from build123d import *

# Parameters (mm, degrees)
SM_BASE_FLANGE_1_DEPTH = 100
CUT_EXTRUDE_1_DEPTH    = 102.727577382
PATTERN_LINEAR_6_COUNT = 4
PATTERN_LINEAR_6_PITCH = 25
SKETCH2_W              = 120.770502754
SKETCH2_H              = 115.80541844
CUT_EXTRUDE1_DEPTH     = 15


# Sheet-metal steps are written as plain solids
with BuildPart() as part:
    # Sketch 1 → Базовая кромка1 (new body)
    with BuildSketch(Plane(origin=(0, 0, 0), x_dir=(0, 0, -1), z_dir=(1, 0, 0))):
        with BuildLine():
            Line((-17.5, 6.5), (-14.5, 6.5))
            ThreePointArc((-14.5, 6.5), (-13.792893219, 6.207106781), (-13.5, 5.5))
            Line((-13.5, 5.5), (-13.5, 2))
            ThreePointArc((-13.5, 2), (-12.914213562, 0.585786438), (-11.5, 0))
            Line((-11.5, 0), (11.5, 0))
            ThreePointArc((11.5, 0), (12.914213562, 0.585786438), (13.5, 2))
            Line((13.5, 2), (13.5, 5.5))
            ThreePointArc((13.5, 5.5), (13.792893219, 6.207106781), (14.5, 6.5))
            Line((14.5, 6.5), (17.5, 6.5))
            Line((17.5, 6.5), (17.5, 7.5))
            Line((17.5, 7.5), (14.5, 7.5))
            ThreePointArc((14.5, 7.5), (13.085786438, 6.914213562), (12.5, 5.5))
            Line((12.5, 5.5), (12.5, 2))
            ThreePointArc((12.5, 2), (12.207106781, 1.292893219), (11.5, 1))
            Line((11.5, 1), (-11.5, 1))
            ThreePointArc((-11.5, 1), (-12.207106781, 1.292893219), (-12.5, 2))
            Line((-12.5, 2), (-12.5, 5.5))
            ThreePointArc((-12.5, 5.5), (-13.085786438, 6.914213562), (-14.5, 7.5))
            Line((-14.5, 7.5), (-17.5, 7.5))
            Line((-17.5, 7.5), (-17.5, 6.5))
        make_face()
    extrude(amount=SM_BASE_FLANGE_1_DEPTH)

    # Эскиз6 → Вырез-Вытянуть1 (cut, through all)
    with BuildSketch(Plane(origin=(0, 1, 0), x_dir=(1, 0, 0), z_dir=(0, 1, 0))):
        with BuildLine():
            Line((6.65, 3.15), (18.35, 3.15))
            ThreePointArc((18.35, 3.15), (21.5, 0), (18.35, -3.15))
            Line((18.35, -3.15), (6.65, -3.15))
            ThreePointArc((6.65, -3.15), (3.5, 0), (6.65, 3.15))
        make_face()
    cut_extrude_1 = extrude(amount=-CUT_EXTRUDE_1_DEPTH, mode=Mode.SUBTRACT)

    # Линейный массив6: Вырез-Вытянуть1 ×4
    with Locations(*[(i * PATTERN_LINEAR_6_PITCH, 0, 0) for i in range(1, PATTERN_LINEAR_6_COUNT)]):
        add(cut_extrude_1, mode=Mode.SUBTRACT)

    # Sketch2 → Cut-Extrude1 (cut)
    with BuildSketch(Plane.ZY):
        with Locations((-11.279080545, 0.592045476)):
            Rectangle(SKETCH2_W, SKETCH2_H)
    extrude(amount=-CUT_EXTRUDE1_DEPTH, mode=Mode.SUBTRACT)


solid = part.part
Geometry check sheet. Reference: the model listing, model coordinates, mm. A direction names the side the tool comes from. Round coordinates to 2 decimals unless told otherwise and drop trailing zeros. Order: outer loops, then holes, each group sorted by start corner. A loop starts at its lowest first (then second) coordinate and runs counter-clockwise, first axis right, second up. Notation, with made-up numbers: (1.25, 85.5) - (38.25, 85.5) arc R16 ccw to (38.25, 111.5) - close; hole circle Ø6 at (44, -38.5). An arc over 180 degrees is marked (long way). One line per question, with ' | ' between items. Start each with the question number.
(1) Sectioned sample at D-D on x = 20.5. Record the cut outline in (y, z).
(2) Thickness scan on L1, parallel to Z at x = 68, y = 4; L2, parallel to Y at x = 85.5, z = 8; L3, parallel to Y at x = 63, z = -14.5. Record the ranges inside material, lowest first. Write a range as [from, to].
(3) Sectioned sample at A-A on z = 0. Record the cut outline in (x, y), and give its area (3 significant figures).
(4) Release check for a two-part mould opening along Z. For faces 1 (the cylindrical face through (78.5, 0.5, 0.1)), 2 (the flat face through (57, 4, -12.5)), 3 (the flat face through (57, 6.5, 16)), 4 (the cylindrical face through (56.9, 0.6, 12.93)) record: released by +Z, released by -Z, zero draft, split by the parting line, or undercut.
(5) Depth check by flat-ended pin: pin 1 Ø1.1 at (x, y) = (35.5, 0.5) entering from +Z; pin 2 Ø1 at (x, z) = (48.5, 13.5) entering from -Y; pin 3 Ø0.5 at (x, y) = (38, 0.5) entering from -Z. Enter the tip coordinate at first touch or a pass-through.
(6) Sectioned sample at C-C on x = 75. Record the cut outline in (y, z).
(7) Access from +Z, -Z, +X, -X, +Y, -Y to the whole of each face (thin tool, end or side, straight path). Record for faces 5 (the flat face through (57, 1, -5)), 6 (the flat face through (57, 4, 13.5)), 7 (the flat face through (57, 4, -13.5)), 8 (the cylindrical face through (96.5, 0.5, -0.1)).
(8) Sectioned sample at B-B on y = 3.5. Record the cut outline in (x, z), and give its area (3 significant figures).
Conclusion:
1) outline: (0, -11.5) arc R2 ccw to (2, -13.5) - (5.5, -13.5) arc R1 cw to (6.5, -14.5) - (6.5, -17.5) - (7.5, -17.5) - (7.5, -14.5) arc R2 ccw to (5.5, -12.5) - (2, -12.5) arc R1 cw to (1, -11.5) - (1, -2.3) - (0, -2.3) - close; (0, 2.3) - (1, 2.3) - (1, 11.5) arc R1 cw to (2, 12.5) - (5.5, 12.5) arc R2 ccw to (7.5, 14.5) - (7.5, 17.5) - (6.5, 17.5) - (6.5, 14.5) arc R1 cw to (5.5, 13.5) - (2, 13.5) arc R2 ccw to (0, 11.5) - close
2) L1: z = [-13.5, -12.5], [12.5, 13.5] | L2: y = [0, 1] | L3: y = [6.5, 7.5]
3) outline: (21.5, 0) - (28.5, 0) - (28.5, 1) - (21.5, 1) - close; (46.5, 0) - (53.5, 0) - (53.5, 1) - (46.5, 1) - close; (71.5, 0) - (78.5, 0) - (78.5, 1) - (71.5, 1) - close; (96.5, 0) - (100, 0) - (100, 1) - (96.5, 1) - close | area: 24.5 mm2
4) face 1: undercut | face 2: undercut | face 3: zero draft | face 4: released by +Z
5) pin 1: stops at z = 13.26 | pin 2: stops at y = 0.68 | pin 3: stops at z = -13.06
6) outline: (0, -11.5) arc R2 ccw to (2, -13.5) - (5.5, -13.5) arc R1 cw to (6.5, -14.5) - (6.5, -17.5) - (7.5, -17.5) - (7.5, -14.5) arc R2 ccw to (5.5, -12.5) - (2, -12.5) arc R1 cw to (1, -11.5) - (1, 11.5) arc R1 cw to (2, 12.5) - (5.5, 12.5) arc R2 ccw to (7.5, 14.5) - (7.5, 17.5) - (6.5, 17.5) - (6.5, 14.5) arc R1 cw to (5.5, 13.5) - (2, 13.5) arc R2 ccw to (0, 11.5) - close
7) face 5: +X, -X, +Y | face 6: +Z, +X, -X, -Y | face 7: -Z, +X, -X, -Y | face 8: +Y, -Y
8) outline: (15, -13.5) - (100, -13.5) - (100, -12.5) - (15, -12.5) - close; (15, 12.5) - (100, 12.5) - (100, 13.5) - (15, 13.5) - close | area: 170 mm2
